Autodesk Inventor part; units mm, degrees
ref_plane "YZ Plane" through (0, 0, 0) normal (1, 0, 0) x (0, 1, 0)
ref_plane "XZ Plane" through (0, 0, 0) normal (0, 1, 0) x (-1, 0, 0)
ref_plane "XY Plane" through (0, 0, 0) normal (0, 0, 1) x (1, 0, 0)
sketch "Sketch1" plane through (0, 0, 0) normal (0, 0, 1) x (1, 0, 0)
  line L0 (0, 0) -> (8, 0)
  line L1 (8, 0) -> (8, 1)
  line L2 (8, 1) -> (1, 1)
  line L3 (1, 1) -> (1, 5)
  line L4 (1, 5) -> (0, 5)
  line L5 (0, 5) -> (0, 0)
  dimension "d0" = 8
  dimension "d1" = 5
  dimension "d2" = 1
  dimension "d8" = 1
extrude "Extrusion1" add sketch "Sketch1" along normal blind 7
sketch "Sketch2" plane through (0, 0, 0) normal (-1, 0, 0) x (0, 0, 1)
  circle A0 centre (3.5, 2.55) radius 1.55
  line L0 (0, 0) -> (7, 0)
  line L1 (7, 5) -> (7, 0)
  dimension "d5" = 3.1
  dimension "d6" = 2.55
  dimension "d7" = 3.5
extrude "Extrusion2" add sketch "Sketch2" along normal blind 2
sketch "Sketch3" plane through (1, 1, 0) normal (0, 1, 0) x (1, 0, 0)
  line L0 (7, 0) -> (7, -7)
  line L1 (7, -7) -> (0, -7)
  point P0 (-1, 0)
  point P1 (3.5, -3.5)
  point P2 (3.5, -7)
  dimension "d11" = 3.5
  dimension "d12" = 3.5
hole "Hole1" at (4.5, 1, 3.5) direction (0, -1, 0) diameter 3.1 end through all
sketch "Sketch4" plane through (1, 1, 0) normal (0, 1, 0) x (1, 0, 0)
  line L0 (3.5, -0.495) -> (6.1024, -1.9975)
  line L1 (6.1024, -1.9975) -> (6.1024, -5.0025)
  line L2 (6.1024, -5.0025) -> (3.5, -6.505)
  line L3 (3.5, -6.505) -> (0.8976, -5.0025)
  line L4 (0.8976, -5.0025) -> (0.8976, -1.9975)
  line L5 (0.8976, -1.9975) -> (3.5, -0.495)
  circle A0 centre (3.5, -3.5) radius 1.55
  point P0 (-1, 0)
  dimension "d20" = 6.01
fillet "Fillet1" radius 3 2 edges at (8, 0.5, 0) (8, 0.5, 7)
extrude "Extrusion3" cut sketch "Sketch4" against normal blind 0.5
chamfer "Chamfer1" distance 3 angle 45 2 edges at (0.5, 5, 7) (0.5, 5, 0)
fillet "Fillet2" radius 3 2 edges at (0.5, 5, 4) (0.5, 5, 3)
properties part number "mocowanie_tofa_CPY1"
Could you check a few things on this model? Use its own coordinates, in mm. A direction names the side the tool comes from. Coordinates: 2 decimals unless noted, no trailing zeros. Write each loop counter-clockwise with the first axis right and the second up, starting at its lowest first coordinate (ties: lowest second). Pieces come first, ordered by that corner, then holes. Notation, with made-up numbers: M 48.25,45 L 100.25,45 A21 ccw 100.25,76 Z; hole C 21,66 d3. An arc over 180 degrees is marked long. Answer as CSV lines item,"result". Start each with the question number.
1) Please list where these lines run through material, in increasing order: line 1 (Z direction, x = 4.5, y = 0.2); line 2 (X direction, y = 0.45, z = 3.5); line 3 (X direction, y = 3.55, z = 2). Write a range as from..to.
2) I want a section at B-B, the plane x = 4.25. Please give me the cut outline in (y, z), and give its area (3 significant figures).
3) For faces 1 (the cylindrical face through (7.1, 0.51, 6.14)), 2 (the flat face through (3, 1, 1)), 3 (the flat face through (3.181, 0.754, 1.257)), which set-ups out of +Z, -Z, +X, -X, +Y, -Y let a thin tool reach every point of the face, with its end or its side?
4) I want a section at C-C, the plane y = 0.7. Please give me the cut outline in (x, z) (1 decimal), and give its area (3 significant figures).
5) For P1, Ø2, axis at x = 3.5, z = 2.5, coming from the +Y side; P2, Ø4, axis at x = 5, z = 2.5, coming from the +Y side; P3, Ø1, axis at y = 2.5, z = 3, coming from the +X side, each with a flat end and sliding along its axis, tell me the tip position at first contact or that it passes through.
6) I want a section at A-A, the plane z = 3.5. Please give me the cut outline in (x, y), and give its area (3 significant figures).
7) I want a section at D-D, the plane y = 2.55. Please give me the cut outline in (x, z).
Data:
1,line 1,"z = 0..1.95, 5.05..7"
1,line 2,"x = 0..2.95, 6.05..8"
1,line 3,"x = 0..1"
2,outline,"M 0,0 L 1,0 L 1,0.64 L 0.5,0.64 L 0.5,1.97 L 0,1.97 Z; M 0,5.03 L 0.5,5.03 L 0.5,6.36 L 1,6.36 L 1,7 L 0,7 Z"
2,area,"2.61 mm^2"
3,face 1,"+Z, +X, +Y, -Y"
3,face 2,"+Z, -Z, +X, +Y"
3,face 3,"+Y"
4,outline,"M 0,0 L 5,0 A3 ccw 8,3 L 8,4 A3 ccw 5,7 L 0,7 Z; hole M 1.9,2 L 4.5,0.5 L 7.1,2 L 7.1,5 L 4.5,6.5 L 1.9,5 Z"
4,area,"28.7 mm^2"
5,P1,"stops at y = 0.5"
5,P2,"stops at y = 1"
5,P3,"stops at x = 1"
6,outline,"M -2,1 L 0,1 L 0,0 L 2.95,0 L 2.95,0.5 L 1.9,0.5 L 1.9,1 L 1,1 L 1,4.26 L 0,4.26 L 0,4.1 L -2,4.1 Z; M 6.05,0 L 8,0 L 8,1 L 7.1,1 L 7.1,0.5 L 6.05,0.5 Z"
6,area,"13.3 mm^2"
7,outline,"M -2,1.95 L 0,1.95 L 0,0.55 L 1,0.55 L 1,6.45 L 0,6.45 L 0,5.05 L -2,5.05 Z"
